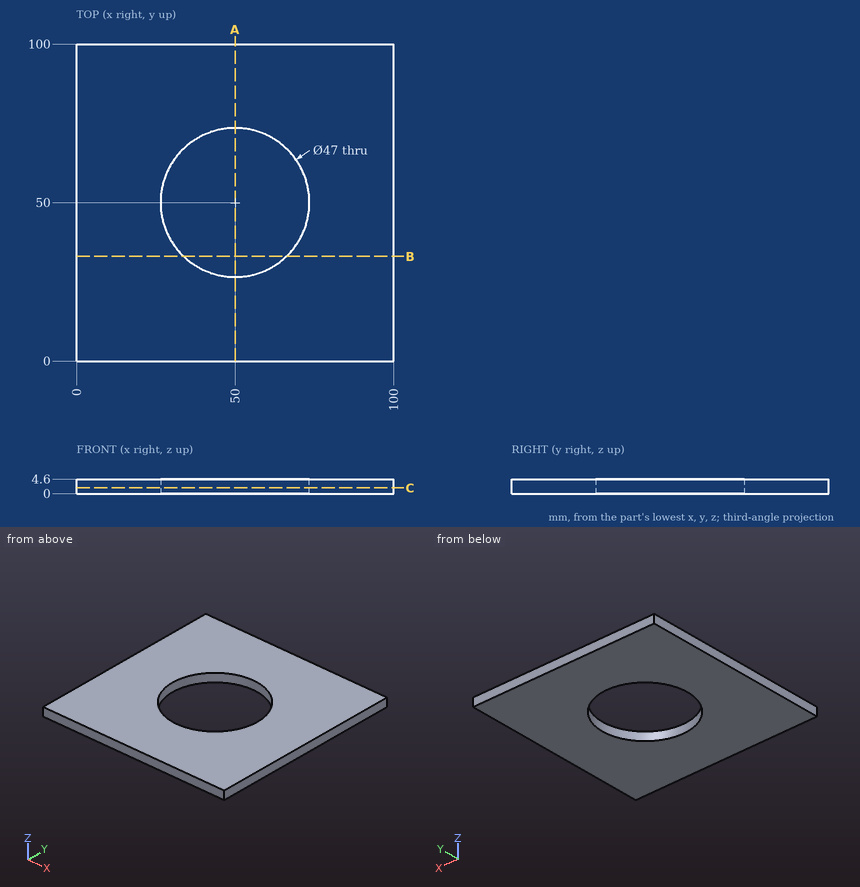
Verification items for this drawing (mm, ordinates from the low corner). Round coordinates to 2 decimals unless told otherwise and drop trailing zeros. Write each loop counter-clockwise with the first axis right and the second up, starting at its lowest first coordinate (ties: lowest second). Pieces come first, ordered by that corner, then holes. Notation, with made-up numbers: M 32,67 L 69,67 A12 cw 69,79 Z; hole C 35,-18.5 d11. An arc over 180 degrees is marked long. Write item = value, one per line. Start each with the question number.
1. Section check A-A, the plane x = 50. Record the cut outline in (y, z).
2. Gauge pin test, flat end, axial feed: pin 1 (8 mm diameter, centred on x = 39.5, y = 72, fed in from -Z). Record the tip position at first contact, or that the pin passes through.
3. Section check C-C, the plane z = 1.8. Record the cut outline in (x, y), then the cut area to 3 significant figures.
4. Scan lines: line 1 (Y direction, x = 50, z = 2.8); line 2 (Y direction, x = 35.5, z = 1.05); line 3 (X direction, y = 68, z = 0.35). Record each from-to range of solid material in increasing order. Write a range as [from, to].
5. Section check B-B, the plane y = 33. Record the cut outline in (x, z), then the cut area to 3 significant figures.
Results found:
q1.outline = M 0,0 L 26.5,0 L 26.5,4.6 L 0,4.6 Z; M 73.5,0 L 100,0 L 100,4.6 L 73.5,4.6 Z
q2.pin_1 = 0
q3.outline = M 0,0 L 100,0 L 100,100 L 0,100 Z; hole C 50,50 d47
q3.area = 8,270 mm^2
q4.line_1 = [0, 26.5], [73.5, 100]
q4.line_2 = [0, 31.51], [68.49, 100]
q4.line_3 = [0, 34.89], [65.11, 100]
q5.outline = M 0,0 L 33.78,0 L 33.78,4.6 L 0,4.6 Z; M 66.22,0 L 100,0 L 100,4.6 L 66.22,4.6 Z
q5.area = 311 mm^2
